Part model, mm, in its own coordinate system. A direction names the side the tool comes from. Round coordinates to 2 decimals unless told otherwise and drop trailing zeros. Order: outer loops, then holes, each group sorted by start corner. A loop starts at its lowest first (then second) coordinate and runs counter-clockwise, first axis right, second up. Notation, with made-up numbers: M 83.5,32 L 97.5,32 A38 cw 97.5,71 Z; hole C -38.5,10 d2. An arc over 180 degrees is marked long. One line per question, with ' | ' between items.
from build123d import *

# Parameters (mm, degrees)
BOSS_EXTRUDE1_DEPTH = 1.5
SKETCH2_R           = 6
BOSS_EXTRUDE2_DEPTH = 8
SKETCH3_R           = 2.764055342
BOSS_EXTRUDE3_DEPTH = 7


with BuildPart() as part:
    # Sketch1 → Boss-Extrude1 (new body)
    with BuildSketch(Plane(origin=(0, 0, 0), x_dir=(1, 0, 0), z_dir=(0, 1, 0))):
        Polygon((-19, 10.5), (19, 10.5), (29, 4.5), (29, -4.5), (19, -10.5), (-19, -10.5), (-29, -4.5), (-29, 4.5), align=None)
    extrude(amount=BOSS_EXTRUDE1_DEPTH)

    # Sketch2 → Boss-Extrude2 (add)
    with BuildSketch(Plane(origin=(0, 1.5, 0), x_dir=(1, 0, 0), z_dir=(0, 1, 0))):
        with Locations(Location((-17, 0, 0), (0, 0, 270))):
            Circle(SKETCH2_R)
    extrude(amount=BOSS_EXTRUDE2_DEPTH)

    # Sketch3 → Boss-Extrude3 (add)
    with BuildSketch(Plane(origin=(0, 1.5, 0), x_dir=(1, 0, 0), z_dir=(0, 1, 0))):
        with Locations(Location((0, 0, 0), (0, 0, 90))):
            Circle(SKETCH3_R)
    extrude(amount=BOSS_EXTRUDE3_DEPTH)


solid = part.part
1) Two-plate mould, pull along X, no slides. Class faces 1 (the face through (-23.93, 0.74, 7.54)), 2 (the face through (-0.83, 4.951, -2.636)), 3 (the face through (23.93, 0.74, -7.54)): released by +X, released by -X, zero draft, split by the parting line, or undercut.
The answers:
face 1: released by -X | face 2: undercut | face 3: released by +X
2) Saw through at C-C (y = 4). List the corners of the cut face in (x, z), plus the area to 3 significant figures.
The answers:
outline: C -17,0 d12; C 0,0 d5.53 | area: 137 mm²
3) Probe line 1 (Y direction, x = 15, z = -2.75); line 2 (X direction, y = 6.75, z = -2.5); line 3 (X direction, y = 2.75, z = -1.75). List the from-to ranges inside material, lowest first. Write a range as [from, to].
The answers:
line 1: y = [0, 1.5] | line 2: x = [-22.45, -11.55], [-1.18, 1.18] | line 3: x = [-22.74, -11.26], [-2.14, 2.14]
4) Saw through at D-D (x = -17). List the corners of the cut face in (y, z), plus the area to 4 significant figures.
The answers:
outline: M 0,-10.5 L 1.5,-10.5 L 1.5,-6 L 9.5,-6 L 9.5,6 L 1.5,6 L 1.5,10.5 L 0,10.5 Z | area: 127.5 mm²
5) Saw through at A-A (x = 0). List the corners of the cut face in (y, z), plus the area to 3 significant figures.
The answers:
outline: M 0,-10.5 L 1.5,-10.5 L 1.5,-2.76 L 8.5,-2.76 L 8.5,2.76 L 1.5,2.76 L 1.5,10.5 L 0,10.5 Z | area: 70.2 mm²
6) Which spindle directions (+Z, -Z, +X, -X, +Y, -Y) get a long thin tool onto all of the face, cutting with end or side? Do faces 4 (the face through (-29, 1, 0)), 5 (the face through (-11.05, 5.44, -0.78)), 6 (the face through (0, 8.5, 0)). Say none if no direction does.
The answers:
face 4: +Z, -Z, -X, +Y, -Y | face 5: +Y | face 6: +Z, -Z, +X, +Y
7) Saw through at B-B (z = 0). List the corners of the cut face in (x, y), plus the area to 3 significant figures.
The answers:
outline: M -29,0 L 29,0 L 29,1.5 L 2.76,1.5 L 2.76,8.5 L -2.76,8.5 L -2.76,1.5 L -11,1.5 L -11,9.5 L -23,9.5 L -23,1.5 L -29,1.5 Z | area: 222 mm²
8) Drop flat-ended pins along their axis: pin 1 (4 mm diameter, centred on x = -3.5, z = 7.5, fed in from +Y); pin 2 (2 mm diameter, centred on x = 2, z = 1, fed in from +Y); pin 3 (2 mm diameter, centred on y = 8, z = 1, fed in from -X). Give the stop position or say it passes through.
The answers:
pin 1: stops at y = 1.5 | pin 2: stops at y = 8.5 | pin 3: stops at x = -23
